```python
from build123d import *

# Parameters (mm, degrees)
F0_R      = 31.75
F1_DEPTH  = 12.7
F2_R      = 7.9375
F2_R_2    = 4.7625
F3_DEPTH  = 12.7
F3_FACE_R = 4.7625
F4_DEPTH  = 25.4
F5_R      = 3.175
F6_DEPTH  = 25.4


with BuildPart() as f1:
    # F0 (on Top) → F1 (new body)
    with BuildSketch(Plane.XY):
        Circle(F0_R)
    extrude(amount=-F1_DEPTH)

    # F2 (on face) → F3 (join)
    with BuildSketch(Plane.XY):
        Circle(F2_R)
        Circle(F2_R_2, mode=Mode.SUBTRACT)
    extrude(amount=F3_DEPTH)

    # F3_face (on face) → F4 (cut)
    with BuildSketch(Plane.XY):
        Circle(F3_FACE_R)
    extrude(amount=-F4_DEPTH, mode=Mode.SUBTRACT)

    # F5 (on face) → F6 (cut)
    with BuildSketch(Plane.XY):
        with Locations((-25.4, 0)):
            Circle(F5_R)
        with Locations((0, -25.4)):
            Circle(F5_R)
        with Locations((25.4, 0)):
            Circle(F5_R)
        with Locations((0, 25.4)):
            Circle(F5_R)
    extrude(amount=-F6_DEPTH, mode=Mode.SUBTRACT)


solid = f1.part
```
Check sheet for the modelled part. Datum: model origin and axes. Units: mm. A direction names the side the tool comes from. Coordinates: 2 decimals unless noted, no trailing zeros. Order: outer loops, then holes, each group sorted by start corner. A loop starts at its lowest first (then second) coordinate and runs counter-clockwise, first axis right, second up. Notation, with made-up numbers: M 40.5,59.25 L 93.5,59.25 A24 ccw 93.5,81.25 Z; hole C 8,66 d1. An arc over 180 degrees is marked long. Write each question's results on one line, items separated by ' | '. Start each with the question number.
1. Cross-section at A-A on y = 25.4. Record the cut outline in (x, z) (3 decimals).
2. Material ranges on probe 1 along X at (y, z) = (1, -2.25); probe 2 along Y at (x, z) = (-0.5, -8.75); probe 3 along Z at (x, y) = (22, -16), recorded low to high.
3. Mould release check, pull along X, two halves, no side actions. Record for faces 1 (the face through (-6.883, -30.995, -6.261)), 2 (the face through (0, -5, 12.7)), 3 (the face through (-22.37, 0.95, -6.26)): +X half, -X half, draft (parallel to the pull), parting line (faces both ways), or undercut.
4. Access from +Z, -Z, +X, -X, +Y, -Y to the whole of each face (thin tool, end or side, straight path). Record for faces 4 (the face through (-1.72, -7.75, 6.26)), 5 (the face through (-0.41, 28.55, -6.26)).
5. Cross-section at B-B on x = 0. State how many separate pieces and enclosed holes the cut face has, and give its area (3 significant figures).
6. Go/stop test with flat-tipped pins: P1, Ø1, axis at x = 5.5, z = -1.5, coming from the -Y side; P2, Ø4, axis at y = 17.5, z = 1.5, coming from the -X side; P3, Ø10, axis at x = 25.4, y = 0, coming from the +Z side. Record where each tip stops, or that it passes through.
Checks:
1) outline: M -19.05,-12.7 L -3.175,-12.7 L -3.175,0 L -19.05,0 Z; M 3.175,-12.7 L 19.05,-12.7 L 19.05,0 L 3.175,0 Z
2) probe 1: x = -31.73 to -28.41, -22.39 to -4.66, 4.66 to 22.39, 28.41 to 31.73 | probe 2: y = -31.75 to -28.54, -22.26 to -4.74, 4.74 to 22.26, 28.54 to 31.75 | probe 3: z = -12.7 to 0
3) face 1: parting line | face 2: draft | face 3: undercut
4) face 4: +Z | face 5: +Z, -Z
5) separate pieces: 4 | enclosed holes: 0 | area: 605 mm²
6) P1: stops at y = -31.35 | P2: stops at x = -27.32 | P3: stops at z = 0
